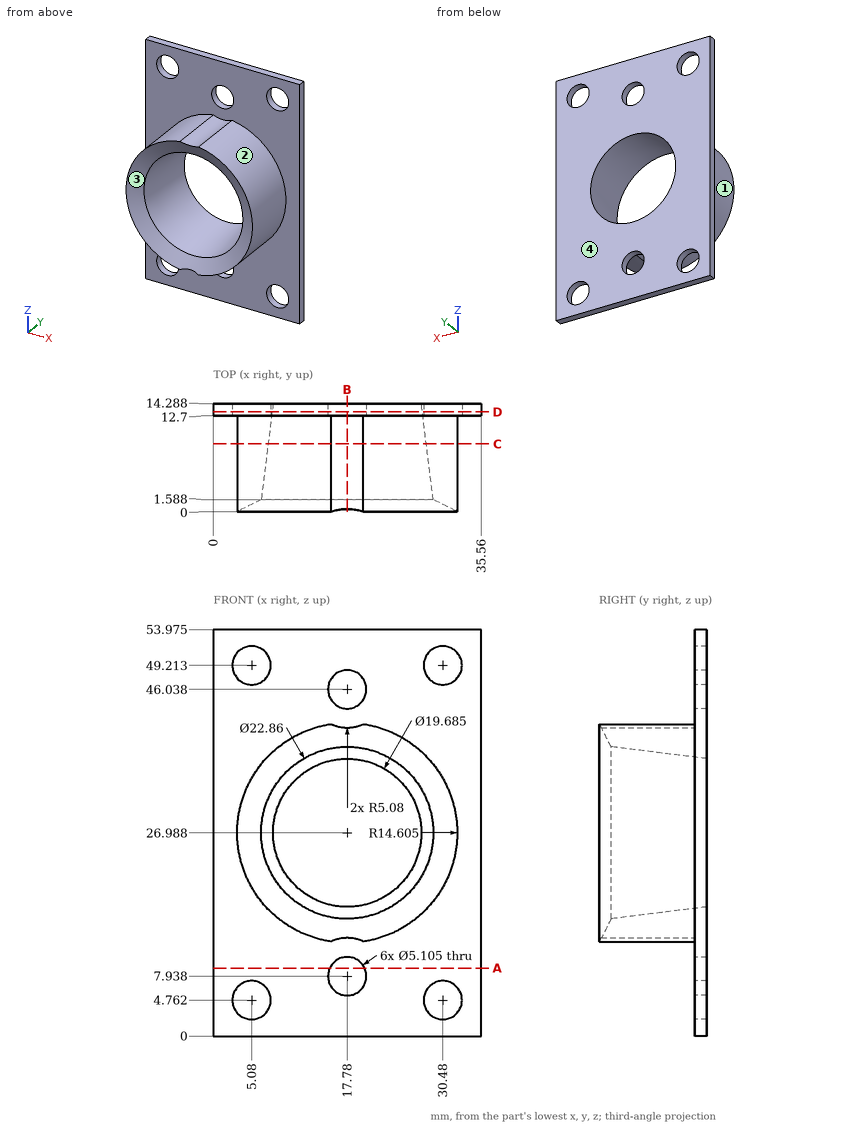
Study the drawing (mm; zero at the part's minimum x, y, z) and answer. Give positions to 0.01 mm unless a question says otherwise; leave off trailing zeros. Loops run counter-clockwise (first coordinate to the right, second up) from the corner with the lowest first, then second, coordinate; pieces in that order, holes last. Notation, with made-up numbers: M 4,84 L 57,84 A24 cw 57,103 Z; hole C 89.5,4 d4. An arc over 180 degrees is marked long. One line per item, written item: value.
1. Section A-A on z = 9 is taken. Determine the outline of the cut face in (x, y).
Found:
outline: M 0,12.7 L 15.46,12.7 L 15.46,14.29 L 0,14.29 Z; M 20.1,12.7 L 35.56,12.7 L 35.56,14.29 L 20.1,14.29 Z
2. Each of these flat-tipped pins is pushed along its axis until it touches: P1, Ø1.5, axis at x = 6, y = 11, coming from the +Z side; P2, Ø1.5, axis at y = 6.5, z = 27, coming from the +X side (1 decimal); P3, Ø1.5, axis at y = 11, z = 19.5, coming from the -X side. Where does it stop, or does it pass through?
Found:
P1: z = 36.56
P2: x = 32.4
P3: x = 4.82
3. For a pull along X with two mould halves and no side action, classify the marked faces 1, 2, 3 and 4 as pulls with the +X half, pulls with the -X half, needs draft (parallel to the pull), parting line crosses it, or undercut.
Found:
face 1: pulls with the -X half
face 2: pulls with the +X half
face 3: undercut
face 4: needs draft
4. Section D-D on y = 13.25 is taken. Determine the outline of the cut face in (x, z) (1 decimal).
Found:
outline: M 0,0 L 35.6,0 L 35.6,54 L 0,54 Z; hole C 5.1,4.8 d5.1; hole C 5.1,49.2 d5.1; hole C 17.8,27 d19.9; hole C 17.8,7.9 d5.1; hole C 17.8,46 d5.1; hole C 30.5,4.8 d5.1; hole C 30.5,49.2 d5.1
5. Section C-C on y = 9 is taken. Determine the outline of the cut face in (x, z) (1 decimal), plus the area to 3 significant figures.
Found:
outline: M 15.6,12.5 A5.1 cw 19.9,12.5 A14.6 ccw 19.9,41.4 A5.1 cw 15.6,41.4 A14.6 ccw Z; hole C 17.8,27 d21
area: 320 mm^2
6. Find the intervals of material crossed by probe 1 along Z at (x, y) = (30.48, 13.55) (1 decimal); probe 2 along X at (y, z) = (13.5, 4) (1 decimal); probe 3 along Z at (x, y) = (17.78, 13.95) (1 decimal), in increasing order.
Found:
probe 1: 0 to 2.2, 7.3 to 46.7, 51.8 to 54
probe 2: 0 to 2.6, 7.5 to 28, 32.9 to 35.6
probe 3: 0 to 5.4, 10.5 to 17.1, 36.9 to 43.5, 48.6 to 54
7. Section B-B on x = 17.78 is taken. Determine the outline of the cut face in (y, z) (1 decimal).
Found:
outline: M 0.3,13 L 12.7,13 L 12.7,10.5 L 14.3,10.5 L 14.3,17.1 L 1.6,15.6 Z; M 0.3,41 L 1.6,38.4 L 14.3,36.8 L 14.3,43.5 L 12.7,43.5 L 12.7,41 Z; M 12.7,0 L 14.3,0 L 14.3,5.4 L 12.7,5.4 Z; M 12.7,48.6 L 14.3,48.6 L 14.3,54 L 12.7,54 Z
